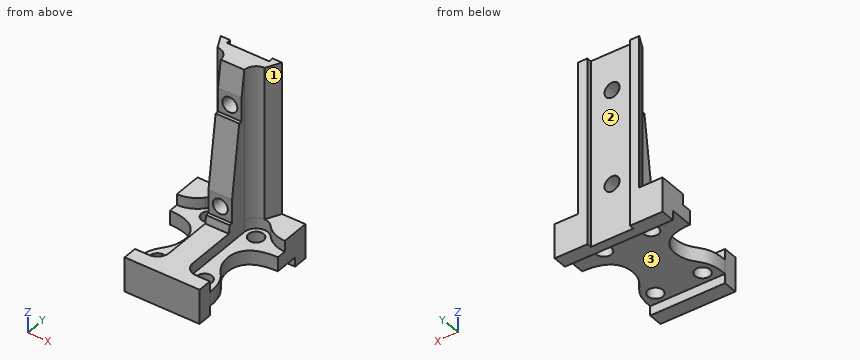
```python
from build123d import *

# Parameters (mm, degrees)
SKETCH_R        = 1.6
PAD_DEPTH       = 5.3
SKETCH001_W     = 22.9
SKETCH001_H     = 3
SKETCH001_W_2   = 15.9
PAD001_DEPTH    = 2
POCKET_DEPTH    = 2.3
PAD002_DEPTH    = 32.3
POCKET001_DEPTH = 10
SKETCH007_W     = 9
SKETCH007_H     = 39.6
POCKET002_DEPTH = 1
SKETCH008_R     = 1.6
POCKET003_DEPTH = 10
SKETCH009_W     = 0.696594
SKETCH009_H     = 5
SKETCH009_W_2   = 0.696595
POCKET004_DEPTH = 5


with BuildPart() as part:
    # Sketch (on Face1 of ReferenceBinder) → Pad (new body)
    with BuildSketch(Plane.XY.offset(8)):
        with BuildLine():
            Line((3, 23), (25.9, 23))
            Line((25.9, 23), (25.9, 15))
            add(Edge.make_bspline(
                [(25.9, 15), (18.45, 15), (18.45, 5), (22.4, 5), (22.4, 0)],
                knots=[0, 0, 0, 0, 0.5, 1, 1, 1, 1], degree=3))
            Line((22.4, 0), (22.4, -3))
            Line((22.4, -3), (6.5, -3))
            Line((6.5, -3), (6.5, 0))
            add(Edge.make_bspline(
                [(3, 15), (10.45, 15), (10.45, 5), (6.5, 5), (6.5, 0)],
                knots=[0, 0, 0, 0, 0.5, 1, 1, 1, 1], degree=3))
            Line((3, 15), (3, 23))
        make_face()
        with Locations((9.45, 17.5)):
            Circle(SKETCH_R, mode=Mode.SUBTRACT)
        with Locations((19.45, 17.5)):
            Circle(SKETCH_R, mode=Mode.SUBTRACT)
        with Locations((19.45, 2.5)):
            Circle(SKETCH_R, mode=Mode.SUBTRACT)
        with Locations((9.45, 2.5)):
            Circle(SKETCH_R, mode=Mode.SUBTRACT)
    extrude(amount=PAD_DEPTH)

    # Sketch001 (on Face1 of ReferenceBinder) → Pad001 (join)
    with BuildSketch(Plane.XY.offset(8)):
        with Locations((14.45, 21.5)):
            Rectangle(SKETCH001_W, SKETCH001_H)
        with Locations((14.45, -1.5)):
            Rectangle(SKETCH001_W_2, SKETCH001_H)
    extrude(amount=-PAD001_DEPTH)

    # Sketch002 (on Face5 of Pad001) → Pocket (cut)
    with BuildSketch(Plane.XY.offset(13.3)):
        with BuildLine():
            ThreePointArc((9.449999, 0), (11.217763, 0.732229), (11.95, 2.499988))
            Line((11.95, 17.5), (11.95, 2.499988))
            ThreePointArc((11.95, 17.5), (10.314365, 19.84582), (7.547701, 19.122116))
            ThreePointArc((3, 17.023415), (5.504303, 17.573395), (7.547701, 19.122116))
            Line((3, 17.023415), (3, 15))
            Line((3, 15), (6.5, 0))
            Line((9.449999, 0), (6.5, 0))
        make_face()
        with BuildLine():
            ThreePointArc((16.95, 2.499988), (17.682233, 0.732233), (19.449988, 0))
            Line((19.449988, 0), (22.4, 0))
            Line((22.4, 0), (25.9, 15))
            Line((25.9, 15), (25.9, 17.023415))
            ThreePointArc((21.352299, 19.122116), (23.395697, 17.573395), (25.9, 17.023415))
            ThreePointArc((21.352299, 19.122116), (18.585635, 19.84582), (16.95, 17.5))
            Line((16.95, 17.5), (16.95, 2.499988))
        make_face()
    extrude(amount=-POCKET_DEPTH, mode=Mode.SUBTRACT)

    # Sketch005 (on Face5 of Pocket) → Pad002 (join)
    with BuildSketch(Plane.XY.offset(13.3)):
        with BuildLine():
            Line((7.95, 23), (20.95, 23))
            Line((20.95, 23), (19.45, 20))
            ThreePointArc((19.45, 20), (17.682233, 19.267767), (16.95, 17.5))
            Line((16.95, 17.5), (16.95, 13))
            Line((16.95, 13), (11.95, 13))
            Line((11.95, 13), (11.95, 17.5))
            ThreePointArc((11.95, 17.5), (11.217767, 19.267767), (9.45, 20))
            Line((9.45, 20), (7.95, 23))
        make_face()
    extrude(amount=PAD002_DEPTH)

    # Sketch006 (on Face39 of Pad002) → Pocket001 (cut)
    with BuildSketch(Plane.YZ.offset(16.95)):
        Polygon((17.5, 45.6), (13, 13.3), (13, 45.6), align=None)
    extrude(amount=-POCKET001_DEPTH, mode=Mode.SUBTRACT)

    # Sketch007 (on Face6 of Pocket001) → Pocket002 (cut)
    with BuildSketch(Plane(origin=(0, 23, 0), x_dir=(-1, 0, 0), z_dir=(0, 1, 0))):
        with Locations((-14.45, 25.8)):
            Rectangle(SKETCH007_W, SKETCH007_H)
    extrude(amount=-POCKET002_DEPTH, mode=Mode.SUBTRACT)

    # Sketch008 (on Face10 of Pocket002) → Pocket003 (cut)
    with BuildSketch(Plane(origin=(0, 22, 0), x_dir=(-1, 0, 0), z_dir=(0, 1, 0))):
        with Locations((-14.45, 37.5)):
            Circle(SKETCH008_R)
        with Locations((-14.45, 17.5)):
            Circle(SKETCH008_R)
    extrude(amount=-POCKET003_DEPTH, mode=Mode.SUBTRACT)

    # Sketch009 (on Face41 of Pocket003) → Pocket004 (cut)
    with BuildSketch(Plane.YZ.offset(16.95)):
        with Locations((16.371517, 37.5)):
            Rectangle(SKETCH009_W, SKETCH009_H)
        with Locations((13.58514, 17.5)):
            Rectangle(SKETCH009_W_2, SKETCH009_H)
    extrude(amount=-POCKET004_DEPTH, mode=Mode.SUBTRACT)


solid = part.part
```
Model file for the job. Use its own axes, mm. Face numbers are marked on the shaded views. A direction names the side the tool comes from. Round coordinates to 2 decimals unless told otherwise and drop trailing zeros. Write each loop counter-clockwise with the first axis right and the second up, starting at its lowest first coordinate (ties: lowest second). Pieces come first, ordered by that corner, then holes. Notation, with made-up numbers: (8, 49.5) - (44, 49.5) arc R26 cw to (44, 87.5) - close; hole circle Ø3 at (-25, 84). An arc over 180 degrees is marked (long way). One line per item, written item: value.
(1) Cut at C-C, the plane x = 14.45. Give the number of separate pieces and of enclosed holes in the cut face, plus the area to 3 significant figures.
Values follow:
separate pieces: 3
enclosed holes: 0
area: 314 mm²
(2) Drop flat-ended pins along their axis: P1, Ø0.6, axis at x = 14.5, y = 13.5, coming from the +Z side; P2, Ø3, axis at x = 23.5, y = 5.5, coming from the +Z side (1 decimal); P3, Ø6, axis at x = 9, y = 1.5, coming from the +Z side; P4, Ø4.5, axis at x = 23.5, y = 14, coming from the +Z side. Give the stop position or say it passes through.
Values follow:
P1: stops at z = 15
P2: passes through
P3: stops at z = 13.3
P4: stops at z = 11
(3) Cut at B-B, the plane z = 37.5. Give the cut face in (x, y), plus the area to 3 significant figures.
Values follow:
outline: (7.95, 23) - (9.45, 20) arc R2.5 cw to (11.95, 17.5) - (11.95, 16.72) - (12.85, 16.72) - (12.85, 22) - (9.95, 22) - (9.95, 23) - close; (16.05, 16.72) - (16.95, 16.72) - (16.95, 17.5) arc R2.5 cw to (19.45, 20) - (20.95, 23) - (18.95, 23) - (18.95, 22) - (16.05, 22) - close
area: 27.7 mm²
(4) Wall check: probe 1 along X at (y, z) = (17.5, 10.4); probe 2 along X at (y, z) = (2.5, 9.05); probe 3 along Z at (x, y) = (22, 16). Give the ranges that are in metal, low to high.
Values follow:
probe 1: x = 3 to 7.85, 11.05 to 17.85, 21.05 to 25.9
probe 2: x = 6.72 to 7.85, 11.05 to 17.85, 21.05 to 22.18
probe 3: z = 8 to 11
(5) 3-axis set-ups, long thin cutter, end or side, ignore diameter. For the marked faces 1, 2 and 3: which of +Z, -Z, +X, -X, +Y, -Y reach the whole face in a straight line?
Values follow:
face 1: +Z, +X, -Y
face 2: +Z, -Z, +Y
face 3: -Z, +X, -X
(6) Cut at D-D, the plane z = 25. Give the cut face in (x, y), plus the area to 3 significant figures.
Values follow:
outline: (7.95, 23) - (9.45, 20) arc R2.5 cw to (11.95, 17.5) - (11.95, 14.63) - (16.95, 14.63) - (16.95, 17.5) arc R2.5 cw to (19.45, 20) - (20.95, 23) - (18.95, 23) - (18.95, 22) - (9.95, 22) - (9.95, 23) - close
area: 55.0 mm²
(7) Cut at A-A, the plane y = 18.5. Give the cut face in (x, z).
Values follow:
outline: (3, 8) - (8.2, 8) - (8.2, 11) - (6.93, 11) - (6.93, 13.3) - (3, 13.3) - close; (10.7, 8) - (18.2, 8) - (18.2, 11) - (17.16, 11) - (17.16, 45.6) - (11.74, 45.6) - (11.74, 11) - (10.7, 11) - close; (20.7, 8) - (25.9, 8) - (25.9, 13.3) - (21.97, 13.3) - (21.97, 11) - (20.7, 11) - close; hole circle Ø3.2 at (14.45, 17.5); hole circle Ø3.2 at (14.45, 37.5)
